The listing builds one solid part. Answer for the finished solid, in the listing's coordinates (mm). Coordinates: 2 decimals unless noted, no trailing zeros. Write each loop counter-clockwise with the first axis right and the second up, starting at its lowest first coordinate (ties: lowest second). Pieces come first, ordered by that corner, then holes. Notation, with made-up numbers: M -18,73.5 L -5,73.5 A11 ccw -5,79.5 Z; hole C 25,79 d3. An arc over 180 degrees is marked long. Answer as a JSON object with one key per item and string values. Group by question number.
from build123d import *

# Parameters (mm, degrees)
SKETCH1_W           = 80
SKETCH1_H           = 60
BOSS_EXTRUDE1_DEPTH = 1
SKETCH2_R           = 3.1
SKETCH2_R_2         = 11.25
CUT_EXTRUDE1_DEPTH  = 10
FILLET1_R           = 1


with BuildPart() as part:
    # Sketch1 → Boss-Extrude1 (new body)
    with BuildSketch(Plane.XY):
        Rectangle(SKETCH1_W, SKETCH1_H)
    extrude(amount=BOSS_EXTRUDE1_DEPTH)

    # Sketch2 → Cut-Extrude1 (cut)
    with BuildSketch(Plane.XY.offset(1)):
        with Locations((-33, 21)):
            Circle(SKETCH2_R)
        with Locations(Location((33, 21, 0), (0, 0, 180))):
            Circle(SKETCH2_R)
        with Locations((33, -21)):
            Circle(SKETCH2_R)
        with Locations(Location((-33, -21, 0), (0, 0, 180))):
            Circle(SKETCH2_R)
        Circle(SKETCH2_R_2)
    extrude(amount=-CUT_EXTRUDE1_DEPTH, mode=Mode.SUBTRACT)

    # Fillet1
    fillet1_edges = [part.edges().sort_by_distance(p)[0] for p in [
        (-40, 30, 0.5),
        (40, 30, 0.5),
        (40, -30, 0.5),
        (-40, -30, 0.5),
    ]]
    fillet(fillet1_edges, radius=FILLET1_R)


solid = part.part
Item 1: A cutting plane is placed at D-D, the plane x = 0. Write down the section's boundary in (y, z).
Item 2: A flat-ended cylindrical pin translates along its axis: pin 1 Ø13.5 at (x, y) = (0, 0) entering from -Z. Find the tip coordinate at first contact, or state that the pin passes through.
Item 3: For a pull along Y with two mould halves and no side action, classify faces 1 (the face through (-9, 7, 1)), 2 (the face through (30.54, -22.886, 0.507)), 3 (the face through (-30.54, -19.114, 0.507)) as +Y half, -Y half, draft (parallel to the pull), parting line (faces both ways), or undercut.
Item 4: A cutting plane is placed at B-B, the plane y = 0. Write down the section's boundary in (x, z).
Item 5: Consider L1, parallel to Y at x = 33, z = 0.45; L2, parallel to X at y = 23.5, z = 0.7; L3, parallel to X at y = -19.5, z = 0.15. Determine where each line is inside the solid, lowest interval first. Write a range as from..to.
Item 6: A cutting plane is placed at C-C, the plane z = 0.45. Write down the section's boundary in (x, y), and give its area (3 significant figures).
Item 7: A cutting plane is placed at A-A, the plane x = 33. Write down the section's boundary in (y, z).
Answer:
{
 "1": {"outline": "M -30,0 L -11.25,0 L -11.25,1 L -30,1 Z; M 11.25,0 L 30,0 L 30,1 L 11.25,1 Z"},
 "2": {"pin 1": "through"},
 "3": {"face 1": "draft", "face 2": "undercut", "face 3": "undercut"},
 "4": {"outline": "M -40,0 L -11.25,0 L -11.25,1 L -40,1 Z; M 11.25,0 L 40,0 L 40,1 L 11.25,1 Z"},
 "5": {"L1": "-30..-24.1, -17.9..17.9, 24.1..30", "L2": "-40..-34.83, -31.17..31.17, 34.83..40", "L3": "-40..-35.71, -30.29..30.29, 35.71..40"},
 "6": {"outline": "M -40,-29 A1 ccw -39,-30 L 39,-30 A1 ccw 40,-29 L 40,29 A1 ccw 39,30 L -39,30 A1 ccw -40,29 Z; hole C -33,-21 d6.2; hole C -33,21 d6.2; hole C 0,0 d22.5; hole C 33,-21 d6.2; hole C 33,21 d6.2", "area": "4,280 mm2"},
 "7": {"outline": "M -30,0 L -24.1,0 L -24.1,1 L -30,1 Z; M -17.9,0 L 17.9,0 L 17.9,1 L -17.9,1 Z; M 24.1,0 L 30,0 L 30,1 L 24.1,1 Z"}
}
